Model file for the job. Use its own axes, mm. Give positions to 0.01 mm unless a question says otherwise; leave off trailing zeros. Loops run counter-clockwise (first coordinate to the right, second up) from the corner with the lowest first, then second, coordinate; pieces in that order, holes last. Notation, with made-up numbers: (-2, 51) - (53, 51) arc R25 ccw to (53, 65) - close; hole circle Ø6 at (62.25, 40.5). An arc over 180 degrees is marked (long way). Use a Markdown table: item, result.
from build123d import *

# Parameters (mm, degrees)
F1_DEPTH = 3.175
F3_DEPTH = 2.413
F4_W     = 20.32
F4_H     = 6.35
F5_DEPTH = 3.3782


with BuildPart() as f1:
    # F0 (on Top) → F1 (new body)
    with BuildSketch(Plane.XY):
        with BuildLine():
            Line((47.28845, 18.161), (-47.28845, 18.161))
            Line((-47.28845, 18.161), (-47.28845, 4.168868))
            ThreePointArc((-47.28845, 4.168868), (-41.500207, -6.479288), (-50.8508, -14.189891))
            Line((-50.8508, -14.189891), (-50.8508, -16.475891))
            ThreePointArc((-50.8508, -16.475891), (-40.986806, -11.161147), (-40.000062, 0))
            Line((-40.000062, 0), (-10.16, 0))
            Line((-10.16, 0), (-10.16, 4.0513))
            Line((-10.16, 4.0513), (10.16, 4.0513))
            Line((10.16, 4.0513), (10.16, 0))
            Line((10.16, 0), (40.000062, 0))
            ThreePointArc((40.000062, 0), (40.986806, -11.161147), (50.8508, -16.475891))
            Line((50.8508, -16.475891), (50.8508, -14.189891))
            ThreePointArc((50.8508, -14.189891), (41.500207, -6.479288), (47.28845, 4.168868))
            Line((47.28845, 4.168868), (47.28845, 18.161))
        make_face()
    extrude(amount=F1_DEPTH)

    # F2 (on face) → F3 (cut)
    with BuildSketch(Plane(origin=(0, 0, 0), x_dir=(1, 0, 0), z_dir=(0, 0, -1))):
        with BuildLine():
            Line((-47.28845, -7.090509), (-47.28845, -14.194691))
            ThreePointArc((-47.28845, -14.194691), (-42.1005, -10.6426), (-47.28845, -7.090509))
        make_face()
        with BuildLine():
            ThreePointArc((47.28845, -7.090509), (42.1005, -10.6426), (47.28845, -14.194691))
            Line((47.28845, -14.194691), (47.28845, -7.090509))
        make_face()
    extrude(amount=-F3_DEPTH, mode=Mode.SUBTRACT)

    # F4 (on face) → F5 (join)
    with BuildSketch(Plane.XY.offset(3.175)):
        with Locations((0, 7.2263)):
            Rectangle(F4_W, F4_H)
    extrude(amount=F5_DEPTH)


solid = f1.part
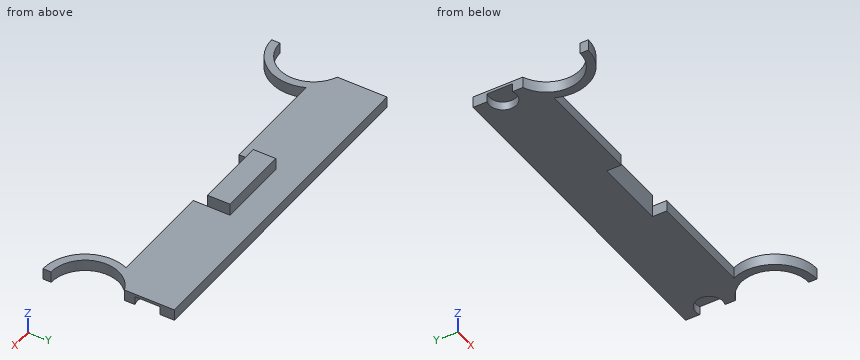
(1) Drill centre lines: probe 1 along Z at (x, y) = (-24, 1) (3 decimals); probe 2 along X at (y, z) = (8, 6.25); probe 3 along X at (y, z) = (0.5, 1). Where is each one in solid material? Low to high. Write a range as [from, to].
Computed:
| item | result |
|---|---|
| probe 1 | [0, 3.175] |
| probe 2 | [-10.16, 10.16] |
| probe 3 | [-42.85, -10.16], [10.16, 42.85] |
(2) Slice it at A-A, the plane y = 2.5. Write the cut outline in (x, z) (3 decimals), plus the area to 3 significant figures.
Computed:
| item | result |
|---|---|
| outline | (-44.575, 0) - (-10.16, 0) - (-10.16, 3.175) - (-44.575, 3.175) - close; (10.16, 0) - (44.575, 0) - (44.575, 3.175) - (10.16, 3.175) - close |
| area | 219 mm² |
(3) Pin check, flat tips, straight feed: P1, Ø3.5, axis at y = 14.5, z = 1.5, coming from the +X side; P2, Ø2.5, axis at y = 7.5, z = 5, coming from the -X side; P3, Ø1.6, axis at x = 24.5, z = 2.5, coming from the -Y side. Stop position of each tip, or through.
Computed:
| item | result |
|---|---|
| P1 | x = 47.29 |
| P2 | x = -10.16 |
| P3 | y = 0 |
(4) Slice it at B-B, the plane x = -3. Write the cut outline in (y, z) (3 decimals), plus the area to 4 significant figures.
Computed:
| item | result |
|---|---|
| outline | (4.051, 0) - (18.161, 0) - (18.161, 3.175) - (10.401, 3.175) - (10.401, 6.553) - (4.051, 6.553) - close |
| area | 66.25 mm² |
(5) Slice it at C-C, the plane y = 8. Write the cut outline in (x, z) (3 decimals).
Computed:
| item | result |
|---|---|
| outline | (-47.288, 2.413) - (-43.166, 2.413) - (-43.166, 0) - (43.166, 0) - (43.166, 2.413) - (47.288, 2.413) - (47.288, 3.175) - (10.16, 3.175) - (10.16, 6.553) - (-10.16, 6.553) - (-10.16, 3.175) - (-47.288, 3.175) - close |
(6) Slice it at D-D, the plane z = 4.5. Write the cut outline in (x, y).
Computed:
| item | result |
|---|---|
| outline | (-10.16, 4.05) - (10.16, 4.05) - (10.16, 10.4) - (-10.16, 10.4) - close |
